Source: CAD feature listing. Evaluate the final solid. Frame: model axes, mm. A direction names the side the tool comes from. Coordinates: 2 decimals unless noted, no trailing zeros. Order: outer loops, then holes, each group sorted by start corner. A loop starts at its lowest first (then second) coordinate and runs counter-clockwise, first axis right, second up.
```python
from build123d import *

# Parameters (mm, degrees)
SKETCH1_W           = 30
SKETCH1_H           = 30
BOSS_EXTRUDE1_DEPTH = 6
BOSS_EXTRUDE4_DEPTH = 20
SKETCH4_W           = 2
SKETCH4_H           = 2
BOSS_EXTRUDE6_DEPTH = 20
SKETCH5_W           = 24
SKETCH5_H           = 6
BOSS_EXTRUDE7_DEPTH = 20
SHELL2_START        = 7
SHELL2_DEPTH        = 23
SHELL2_START_2      = 1
SHELL2_2_DEPTH      = 4
SHELL2_START_3      = 5
SHELL2_3_OUTLINE_W  = 29
SHELL2_3_OUTLINE_H  = 4
SHELL2_3_DEPTH      = 2
SKETCH7_W           = 23
SKETCH7_H           = 1
BOSS_EXTRUDE8_DEPTH = 5
SKETCH9_W           = 1.075143629
SKETCH9_H           = 23
BOSS_EXTRUDE9_DEPTH = 5
SKETCH10_W          = 4
SKETCH10_H          = 23
CUT_EXTRUDE1_DEPTH  = 10
SKETCH11_W          = 23
SKETCH11_H          = 4
CUT_EXTRUDE2_DEPTH  = 10


# Read off the part's stored shape, not the designer's step: Shell2
with BuildPart() as part:
    # Sketch1 → Boss-Extrude1 (new body)
    with BuildSketch(Plane.XY):
        with Locations((15, 15)):
            Rectangle(SKETCH1_W, SKETCH1_H)
    extrude(amount=BOSS_EXTRUDE1_DEPTH)

    # Sketch2 → Boss-Extrude4 (add)
    with BuildSketch(Plane.XY.offset(6)):
        Polygon((5, 6), (6, 6), (6, 30), (0, 30), (0, 6), align=None)
    extrude(amount=BOSS_EXTRUDE4_DEPTH)

    # Sketch4 → Boss-Extrude6 (add)
    with BuildSketch(Plane.XY.offset(6)):
        with Locations((5, 5)):
            Rectangle(SKETCH4_W, SKETCH4_H)
    extrude(amount=BOSS_EXTRUDE6_DEPTH)

    # Sketch5 → Boss-Extrude7 (add)
    with BuildSketch(Plane.XY.offset(6)):
        with Locations((18, 3)):
            Rectangle(SKETCH5_W, SKETCH5_H)
    extrude(amount=BOSS_EXTRUDE7_DEPTH)

    # Shell2 outline → Shell2 (cut)
    with BuildSketch(Plane(origin=(0, 0, 0), x_dir=(1, 0, 0), z_dir=(0, 1, 0)).offset(SHELL2_START)):
        Polygon((5, -5), (30, -5), (30, -1), (1, -1), (1, -25), (5, -25), align=None)
    extrude(amount=SHELL2_DEPTH, mode=Mode.SUBTRACT)

    # Shell2 2 outline → Shell2 2 (cut)
    with BuildSketch(Plane(origin=(0, 0, 0), x_dir=(1, 0, 0), z_dir=(0, 1, 0)).offset(SHELL2_START_2)):
        Polygon((7, -5), (7, -25), (30, -25), (30, -1), (1, -1), (1, -5), align=None)
    extrude(amount=SHELL2_2_DEPTH, mode=Mode.SUBTRACT)

    # Shell2 3 outline → Shell2 3 (cut)
    with BuildSketch(Plane(origin=(0, 0, 0), x_dir=(1, 0, 0), z_dir=(0, 1, 0)).offset(SHELL2_START_3)):
        with Locations((15.5, -3)):
            Rectangle(SHELL2_3_OUTLINE_W, SHELL2_3_OUTLINE_H)
    extrude(amount=SHELL2_3_DEPTH, mode=Mode.SUBTRACT)

    # Sketch7 → Boss-Extrude8 (add)
    with BuildSketch(Plane.XZ.offset(-5)):
        with Locations((18.5, 5.5)):
            Rectangle(SKETCH7_W, SKETCH7_H)
    extrude(amount=BOSS_EXTRUDE8_DEPTH)

    # Sketch9 → Boss-Extrude9 (add)
    with BuildSketch(Plane.ZY.offset(-5)):
        with Locations((5.537571814, 18.5)):
            Rectangle(SKETCH9_W, SKETCH9_H)
    extrude(amount=BOSS_EXTRUDE9_DEPTH)

    # Sketch10 → Cut-Extrude1 (cut)
    with BuildSketch(Plane.XY.offset(26)):
        with Locations((3, 18.5)):
            Rectangle(SKETCH10_W, SKETCH10_H)
    extrude(amount=-CUT_EXTRUDE1_DEPTH, mode=Mode.SUBTRACT)

    # Sketch11 → Cut-Extrude2 (cut)
    with BuildSketch(Plane.XY.offset(26)):
        with Locations((18.5, 3)):
            Rectangle(SKETCH11_W, SKETCH11_H)
    extrude(amount=-CUT_EXTRUDE2_DEPTH, mode=Mode.SUBTRACT)


solid = part.part
```
Q1. Section query A-A on y = 28. Output: boundary loops of the cut face in (x, z), plus the area to 3 significant figures.
Solutions:
outline: (0, 0) - (30, 0) - (30, 1) - (1, 1) - (1, 5) - (30, 5) - (30, 6) - (6, 6) - (6, 26) - (5, 26) - (5, 6.08) - (1, 6.08) - (1, 26) - (0, 26) - close
area: 104 mm2
Q2. Material intervals for line 1 along Y through (x, z) = (15.25, 23), sorted ascending.
Solutions:
line 1: y = 0 to 1, 5 to 6
Q3. Section query B-B on x = 2. Output: boundary loops of the cut face in (y, z), plus the area to 3 significant figures.
Solutions:
outline: (0, 0) - (30, 0) - (30, 1) - (1, 1) - (1, 5) - (30, 5) - (30, 6.08) - (7, 6.08) - (7, 26) - (6, 26) - (6, 6) - (0, 6) - close
area: 85.7 mm2
Q4. Section query D-D on x = 9.5. Output: boundary loops of the cut face in (y, z), plus the area to 3 significant figures.
Solutions:
outline: (0, 0) - (30, 0) - (30, 1) - (1, 1) - (1, 5) - (30, 5) - (30, 6) - (6, 6) - (6, 26) - (5, 26) - (5, 6) - (1, 6) - (1, 26) - (0, 26) - close
area: 104 mm2
Q5. Set-up query: faces 1 (the flat face through (4, 5, 16)), 2 (the flat face through (5, 18, 16)), 3 (the flat face through (18, 18, 6)), 4 (the flat face through (18, 5, 16)), 5 (the flat face through (15, 1, 3)). Return all of +Z, -Z, +X, -X, +Y, -Y with unobstructed straight access to the full face (end or side cutting, diameter ignored); none if empty.
Solutions:
face 1: +Z, -X, -Y
face 2: +Z, +Y
face 3: +Z, +X, +Y
face 4: +Z, +X
face 5: +X, +Y
Q6. Section query C-C on z = 24.25. Output: boundary loops of the cut face in (x, y), plus the area to 3 significant figures.
Solutions:
outline: (0, 6) - (4, 6) - (4, 4) - (6, 4) - (6, 0) - (30, 0) - (30, 1) - (7, 1) - (7, 5) - (30, 5) - (30, 6) - (6, 6) - (6, 30) - (5, 30) - (5, 7) - (1, 7) - (1, 30) - (0, 30) - close
area: 108 mm2
Q7. Pin query (flat end, axial travel): P1, Ø1.2, axis at x = 3.5, z = 16.5, coming from the +Y side; P2, Ø6, axis at y = 14.5, z = 15.5, coming from the +X side; P3, Ø8.5, axis at x = 22.5, y = 20.5, coming from the +Z side. Return the tip coordinate at first contact, or that it passes through.
Solutions:
P1: stops at y = 7
P2: stops at x = 6
P3: stops at z = 6
Q8. Pull-direction query (Z, two-part tool) for faces 6 (the flat face through (1, 18, 16)), 7 (the flat face through (3, 18, 6.075)), 8 (the flat face through (15, 15, 5)); classes: pulls with the +Z half, pulls with the -Z half, needs draft (parallel to the pull), parting line crosses it, or undercut.
Solutions:
face 6: needs draft
face 7: pulls with the +Z half
face 8: undercut
